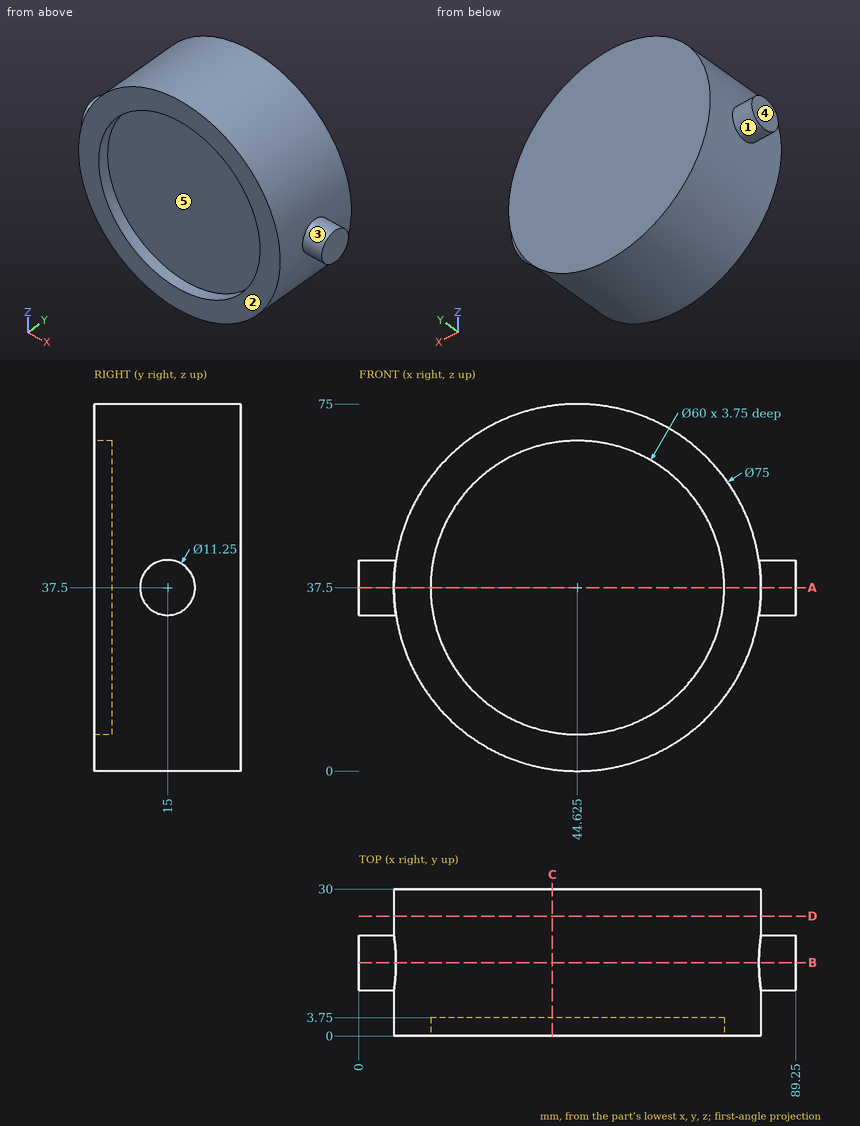
Study the drawing (mm; zero at the part's minimum x, y, z) and answer. A direction names the side the tool comes from. Give positions to 0.01 mm unless a question says otherwise; leave off trailing zeros. Order: outer loops, then holes, each group sorted by start corner. A loop starts at its lowest first (then second) coordinate and runs counter-clockwise, first axis right, second up. Notation, with made-up numbers: M 9,71.5 L 67,71.5 A18 ccw 67,98.5 Z; hole C 48.5,72 d4. An arc over 180 degrees is marked long. Put each result on its own line as item: value. Start each with the question number.
Item 1: The part is cut by section D-D, the plane y = 24.5. Determine the outline of the cut face in (x, z) (3 decimals), and give its area (3 significant figures).
Item 2: The part is cut by section C-C, the plane x = 39.5. Determine the outline of the cut face in (y, z), and give its area (3 significant figures).
Item 3: Flat-ended cylindrical pins translate along their axes: P1, Ø4, axis at x = 36, z = 61.5, coming from the -Y side; P2, Ø8, axis at x = 57, y = 6, coming from the -Z side; P3, Ø6, axis at x = 25.5, y = 21, coming from the +Z side. Find the tip coordinate at first contact, or state that the pin passes through.
Item 4: Which of the six approach directions +Z, -Z, +X, -X, +Y, -Y give full straight-line access (tool end or side, diameter ignored) to the marked faces 1 and 2?
Item 5: The part is cut by section A-A, the plane z = 37.5. Determine the outline of the cut face in (x, y) (3 decimals), and give its area (3 significant figures).
Item 6: Find the intervals of material crossed by line 1 along X through (y, z) = (2.8, 37.5) (3 decimals); line 2 along Y through (x, z) = (25, 19); line 3 along Z through (x, y) = (24.5, 6.5), in increasing order.
Item 7: For a pull along X with two mould halves and no side action, classify the marked faces 3, 4 and 5 as +X half, -X half, draft (parallel to the pull), parting line (faces both ways), or undercut.
Item 8: The part is cut by section B-B, the plane y = 15. Determine the outline of the cut face in (x, z) (3 decimals).
Answer key:
1. outline: C 44.625,37.5 d75
1. area: 4,420 mm²
2. outline: M 0,0.35 L 30,0.35 L 30,74.65 L 0,74.65 L 0,67.06 L 3.75,67.06 L 3.75,7.94 L 0,7.94 Z
2. area: 2,010 mm²
3. P1: stops at y = 3.75
3. P2: stops at z = 0.95
3. P3: stops at z = 71.36
4. face 1: -X
4. face 2: +Z, -Z, +X, -X, -Y
5. outline: M 0,9.375 L 7.125,9.375 L 7.125,0 L 14.625,0 L 14.625,3.75 L 74.625,3.75 L 74.625,0 L 82.125,0 L 82.125,9.375 L 89.25,9.375 L 89.25,20.625 L 82.125,20.625 L 82.125,30 L 7.125,30 L 7.125,20.625 L 0,20.625 Z
5. area: 2,190 mm²
6. line 1: x = 7.125 to 14.625, 74.625 to 82.125
6. line 2: y = 3.75 to 30
6. line 3: z = 5.86 to 69.14
7. face 3: draft
7. face 4: -X half
7. face 5: undercut
8. outline: M 0,31.875 L 7.549,31.875 A37.5 ccw 81.701,31.875 L 89.25,31.875 L 89.25,43.125 L 81.701,43.125 A37.5 ccw 7.549,43.125 L 0,43.125 Z
